Print and shaded views of the part. All mm, measured from the part's lowest x, y and z. A direction names the side the tool comes from. Round coordinates to 2 decimals unless told otherwise and drop trailing zeros. Order: outer loops, then holes, each group sorted by start corner. A loop starts at its lowest first (then second) coordinate and runs counter-clockwise, first axis right, second up. Notation, with made-up numbers: M 42.25,58 L 100.25,58 A26 ccw 100.25,80 Z; hole C 9,65.25 d2. An arc over 180 degrees is marked long. Use CSV: the item, a comma, the result in double quotes.
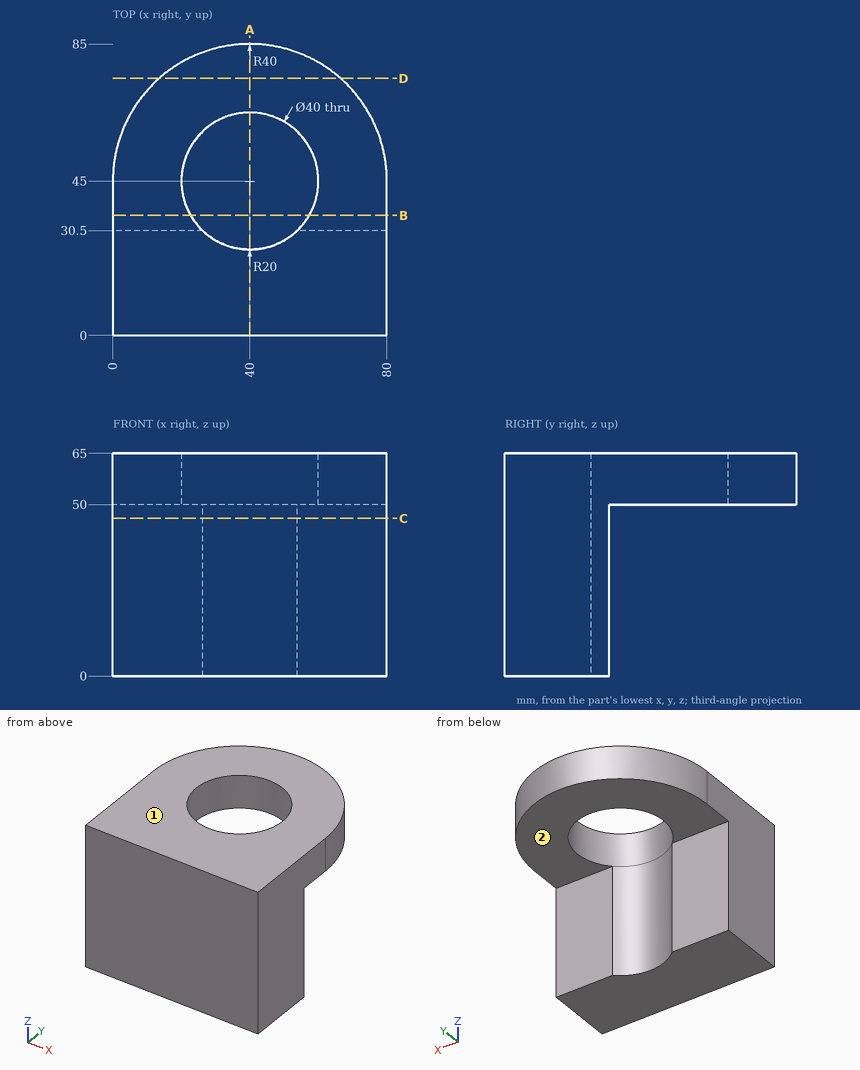
(1) Cut at D-D, the plane y = 75. Give the cut face in (x, z).
Answer block:
outline,"M 13.54,50 L 66.46,50 L 66.46,65 L 13.54,65 Z"
(2) Cut at A-A, the plane x = 40. Give the cut face in (y, z), and give its area (4 significant figures).
Answer block:
outline,"M 0,0 L 25,0 L 25,65 L 0,65 Z; M 65,50 L 85,50 L 85,65 L 65,65 Z"
area,"1,925 mm²"
(3) Cut at B-B, the plane y = 35. Give the cut face in (x, z), and give its area (3 significant figures).
Answer block:
outline,"M 0,50 L 22.68,50 L 22.68,65 L 0,65 Z; M 57.32,50 L 80,50 L 80,65 L 57.32,65 Z"
area,"680 mm²"
(4) Cut at C-C, the plane z = 46. Give the cut face in (x, y), and give its area (3 significant figures).
Answer block:
outline,"M 0,0 L 80,0 L 80,30.5 L 53.77,30.5 A20 cw 26.23,30.5 L 0,30.5 Z"
area,"2,340 mm²"
(5) Tool access for the marked faces 1 and 2: list every direction of +Z, -Z, +X, -X, +Y, -Y with a clear straight run to the whole face (end or side of a thin tool).
Answer block:
face 1,"+Z, +X, -X, +Y, -Y"
face 2,"-Z, +X, -X, +Y"
(6) Wall check: line 1 (X direction, y = 45, z = 59.75); line 2 (Y direction, x = 40, z = 60.75); line 3 (Y direction, x = 68, z = 8.5). Give the ranges that are in metal, low to high. Write a range as from..to.
Answer block:
line 1,"x = 0..20, 60..80"
line 2,"y = 0..25, 65..85"
line 3,"y = 0..30.5"
(7) Drop flat-ended pins along their axis: pin 1 (10 mm diameter, centred on x = 31.5, z = 17.5, fed in from -Y); pin 2 (24 mm diameter, centred on x = 40, y = 45, fed in from -Z); pin 3 (5 mm diameter, centred on x = 24, z = 37.5, fed in from +Y); pin 4 (5 mm diameter, centred on y = 61.5, z = 50, fed in from +X). Give the stop position or say it passes through.
Answer block:
pin 1,"stops at y = 0"
pin 2,"passes through"
pin 3,"stops at y = 30.5"
pin 4,"stops at x = 77.47"
